Design review of the part shown in the three views and the two pictorial views. Dimensions are in mm from the part's minimum x, y and z. Give positions to 0.01 mm unless a question says otherwise; leave off trailing zeros. Write each loop counter-clockwise with the first axis right and the second up, starting at its lowest first coordinate (ties: lowest second). Pieces come first, ordered by that corner, then holes. Notation, with made-up numbers: (-33.5, 47.5) -> (-25.5, 47.5) arc R13 cw to (-25.5, 55.5) -> close; hole circle Ø5 at (86, -16). An arc over 180 degrees is marked (long way). Return JSON: item names as keys, results as strings. Group by question number.
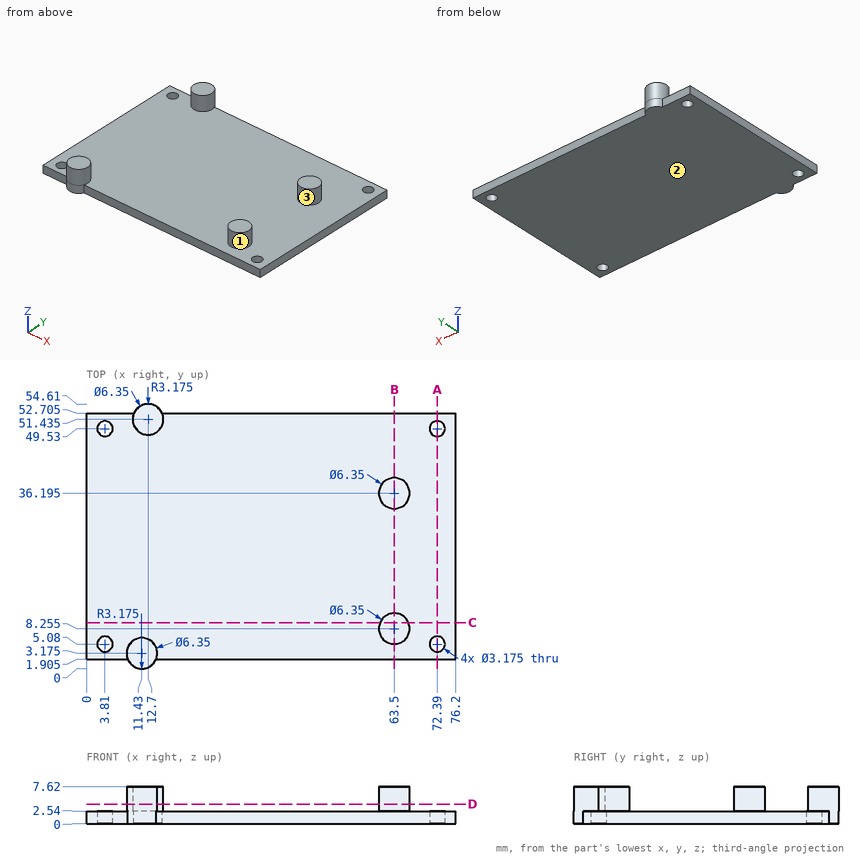
Q1. Mouldability with a two-part tool opening along X and no side actions: class the marked faces 1, 2 and 3 as +X half, -X half, draft (parallel to the pull), parting line (faces both ways), or undercut.
Q2. For L1, parallel to Y at x = 72.39, z = 0.75 (1 decimal); L2, parallel to Z at x = 68, y = 14; L3, parallel to Y at x = 51, z = 2.5 (3 decimals), list the stretches that pass through material, from the lowest coordinate up. Write a range as from..to.
Q3. Take a section at A-A, the plane x = 72.39. Give the boundary of the cut face in (y, z) (1 decimal), plus the area to 3 significant figures.
Q4. Take a section at B-B, the plane x = 63.5. Give the boundary of the cut face in (y, z) (3 decimals).
Q5. Take a section at D-D, the plane z = 4. Give the boundary of the cut face in (x, y) (3 decimals).
Q6. Insertion check: pin 1 (6 mm diameter, centred on x = 35.5, y = 19, fed in from +Z); pin 2 (0.8 mm diameter, centred on x = 6, z = 1.5, fed in from -Y) (3 decimals); pin 3 (3 mm diameter, centred on x = 57, z = 2, fed in from +Y) (3 decimals); pin 4 (2.5 mm diameter, centred on x = 72.39, y = 49.53, fed in from -Z). Each pin has a flat end and moves straight along its axis. Give the tip position at first contact, or say it passes through.
Q7. Take a section at C-C, the plane y = 9.5. Give the boundary of the cut face in (x, z), plus the area to 3 significant figures.
Final values:
{
 "1": {"face 1": "undercut", "face 2": "draft", "face 3": "parting line"},
 "2": {"L1": "y = 1.9..3.5, 6.7..47.9, 51.1..52.7", "L2": "z = 0..2.54", "L3": "y = 1.905..52.705"},
 "3": {"outline": "(1.9, 0) -> (3.5, 0) -> (3.5, 2.5) -> (1.9, 2.5) -> close; (6.7, 0) -> (47.9, 0) -> (47.9, 2.5) -> (6.7, 2.5) -> close; (51.1, 0) -> (52.7, 0) -> (52.7, 2.5) -> (51.1, 2.5) -> close", "area": "113 mm²"},
 "4": {"outline": "(1.905, 0) -> (52.705, 0) -> (52.705, 2.54) -> (39.37, 2.54) -> (39.37, 7.62) -> (33.02, 7.62) -> (33.02, 2.54) -> (11.43, 2.54) -> (11.43, 7.62) -> (5.08, 7.62) -> (5.08, 2.54) -> (1.905, 2.54) -> close"},
 "5": {"outline": "circle Ø6.35 at (11.43, 3.175); circle Ø6.35 at (12.7, 51.435); circle Ø6.35 at (63.5, 8.255); circle Ø6.35 at (63.5, 36.195)"},
 "6": {"pin 1": "stops at z = 2.54", "pin 2": "stops at y = 1.905", "pin 3": "stops at y = 52.705", "pin 4": "passes through"},
 "7": {"outline": "(0, 0) -> (76.2, 0) -> (76.2, 2.54) -> (66.42, 2.54) -> (66.42, 7.62) -> (60.58, 7.62) -> (60.58, 2.54) -> (0, 2.54) -> close", "area": "223 mm²"}
}
